Source: CAD feature listing. Evaluate the final solid. Frame: model axes, mm. Give positions to 0.01 mm unless a question says otherwise; leave off trailing zeros. Order: outer loops, then holes, each group sorted by start corner. A loop starts at its lowest first (then second) coordinate and runs counter-clockwise, first axis right, second up.
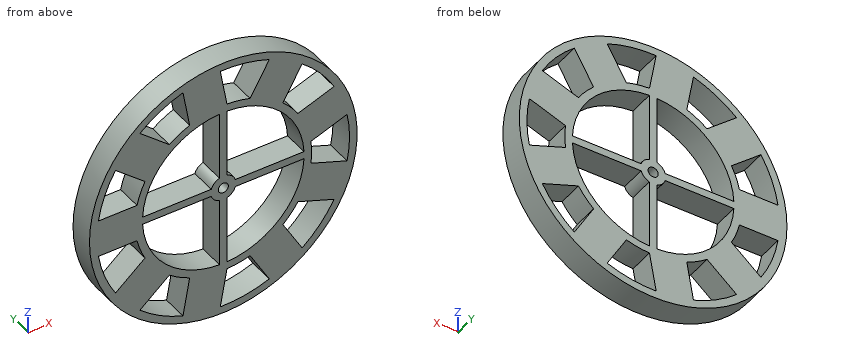
Autodesk Inventor part; units mm, degrees
ref_plane "YZ Plane" through (0, 0, 0) normal (1, 0, 0) x (0, 1, 0)
ref_plane "XZ Plane" through (0, 0, 0) normal (0, 1, 0) x (-1, 0, 0)
ref_plane "XY Plane" through (0, 0, 0) normal (0, 0, 1) x (1, 0, 0)
sketch "Sketch1" plane through (0, 0, 0) normal (0, 1, 0) x (-1, 0, 0)
  circle A0 centre (0, 0) radius 50
  circle A1 centre (0, 0) radius 35
  line L0 (49.4343, 7.5) -> (34.187, 7.5)
  line L1 (49.4343, -7.5) -> (34.187, -7.5)
  line L2 (41.8106, 7.5) -> (41.8106, -7.5) construction
  circle A2 centre (0, 0) radius 32
  line L3 (34.187, 7.5) -> (34.187, -7.5)
  line L4 (49.4343, 7.5) -> (49.4343, -7.5)
  line L5 (21.3678, 27.7203) -> (31.0097, 16.2296)
  line L6 (42.6898, 26.0304) -> (31.0097, 16.2296)
  line L7 (33.048, 37.5211) -> (42.6898, 26.0304)
  line L8 (33.048, 37.5211) -> (21.3678, 27.7203)
  line L9 (-1.4496, 34.97) -> (13.3226, 32.3652)
  line L10 (15.9702, 47.3809) -> (13.3226, 32.3652)
  line L11 (1.1981, 49.9856) -> (15.9702, 47.3809)
  line L12 (1.1981, 49.9856) -> (-1.4496, 34.97)
  line L13 (-23.5887, 25.8568) -> (-10.5983, 33.3568)
  line L14 (-18.222, 46.5614) -> (-10.5983, 33.3568)
  line L15 (-31.2123, 39.0614) -> (-18.222, 46.5614)
  line L16 (-31.2123, 39.0614) -> (-23.5887, 25.8568)
  line L17 (-34.6904, 4.6449) -> (-29.5601, 18.7403)
  line L18 (-43.8879, 23.9552) -> (-29.5601, 18.7403)
  line L19 (-49.0182, 9.8598) -> (-43.8879, 23.9552)
  line L20 (-49.0182, 9.8598) -> (-34.6904, 4.6449)
  line L21 (-29.5601, -18.7403) -> (-34.6904, -4.6449)
  line L22 (-49.0182, -9.8598) -> (-34.6904, -4.6449)
  line L23 (-43.8879, -23.9552) -> (-49.0182, -9.8598)
  line L24 (-43.8879, -23.9552) -> (-29.5601, -18.7403)
  line L25 (-10.5983, -33.3568) -> (-23.5887, -25.8568)
  line L26 (-31.2123, -39.0614) -> (-23.5887, -25.8568)
  line L27 (-18.222, -46.5614) -> (-31.2123, -39.0614)
  line L28 (-18.222, -46.5614) -> (-10.5983, -33.3568)
  line L29 (13.3226, -32.3652) -> (-1.4496, -34.97)
  line L30 (1.1981, -49.9856) -> (-1.4496, -34.97)
  line L31 (15.9702, -47.3809) -> (1.1981, -49.9856)
  line L32 (15.9702, -47.3809) -> (13.3226, -32.3652)
  line L33 (31.0097, -16.2296) -> (21.3678, -27.7203)
  line L34 (33.048, -37.5211) -> (21.3678, -27.7203)
  line L35 (42.6898, -26.0304) -> (33.048, -37.5211)
  line L36 (42.6898, -26.0304) -> (31.0097, -16.2296)
  circle A3 centre (0, 0) radius 53
  circle A4 centre (0, 0) radius 2
  circle A5 centre (0, 0) radius 5
  line L37 (1.5, -31.9648) -> (1.5, -4.7697)
  line L38 (-1.5, -31.9648) -> (-1.5, -4.7697)
  line L39 (1.5, -18.3673) -> (-1.5, -18.3673) construction
  line L40 (-31.9648, -1.5) -> (-4.7697, -1.5)
  line L41 (-4.7697, 1.5) -> (-31.9648, 1.5)
  line L42 (1.5, 31.9648) -> (1.5, 4.7697)
  line L43 (-1.5, 4.7697) -> (-1.5, 31.9648)
  line L44 (4.7697, -1.5) -> (31.9648, -1.5)
  line L45 (4.7697, 1.5) -> (31.9648, 1.5)
  line L46 (18.3673, -1.5) -> (18.3673, 1.5) construction
  line L47 (-1.5, 18.3673) -> (1.5, 18.3673) construction
  line L48 (-18.3673, 1.5) -> (-18.3673, -1.5) construction
  point P0 (41.8106, 0)
  point P1 (36.8497, 21.13)
  point P2 (27.2079, 32.6207)
  point P3 (14.6464, 39.8731)
  point P4 (-0.1257, 42.4778)
  point P5 (-14.4101, 39.9591)
  point P6 (-27.4005, 32.4591)
  point P7 (-36.724, 21.3478)
  point P8 (-41.8543, 7.2524)
  point P9 (-41.8543, -7.2524)
  point P10 (-36.724, -21.3478)
  point P11 (-27.4005, -32.4591)
  point P12 (-14.4101, -39.9591)
  point P13 (-0.1257, -42.4778)
  point P14 (14.6464, -39.8731)
  point P15 (27.2079, -32.6207)
  point P16 (36.8497, -21.13)
  point P17 (0, -18.3673)
  point P18 (-34.6904, -4.6449)
  dimension "d0" = 100
  dimension "d1" = 15
  dimension "d2" = 15
  dimension "d3" = 3
  dimension "d6" = 360
  dimension "d8" = 3
  dimension "d9" = 4
  dimension "d11" = 3
  dimension "d12" = 3
  dimension "d13" = 3
  dimension "d14" = 3
extrude "Extrusion1" add sketch "Sketch1" along normal blind 10 contours A0 L4 | L4 L1 A1 L0 | L7 A0 | L6 A1 L8 L7 | L3 A1 L33 L29 L25 L21 L17 L13 L9 L5 | A1 L3 | A0 L35 | L35 L34 A1 L36 | L5 A1 | A1 L33 | L11 A0 | L10 A1 L12 L11 | A0 L31 | L31 L30 A1 L32 | L9 A1 | A1 L29 | L15 A0 | L14 A1 L16 L15 | A0 L27 | L27 L26 A1 L28 | L13 A1 | A1 L25 | L19 A0 | L18 A1 L20 L19 | A0 L23 | L23 L22 A1 L24 | L17 A1 | A1 L21 | A2 L44 A5 L45 | L42 A5 L43 A2 | A5 | A2 L38 A5 L37 | L41 A5 L40 A2 | A3 | A4
hole "Hole1" at (0, 0, 0) direction (0, 1, 0) diameter 4 end through all
properties part number "Rueda_SENSORVEL_3DPrint"
1) Section query C-C on x = -19. Output: boundary loops of the cut face in (y, z), and give its area (3 significant figures).
Checks:
outline: (0, -49.48) - (10, -49.48) - (10, -46.25) - (0, -46.25) - close; (0, -29.39) - (10, -29.39) - (10, -25.75) - (0, -25.75) - close; (0, -1.5) - (10, -1.5) - (10, 1.5) - (0, 1.5) - close; (0, 25.75) - (10, 25.75) - (10, 29.39) - (0, 29.39) - close; (0, 46.25) - (10, 46.25) - (10, 49.48) - (0, 49.48) - close
area: 167 mm2
2) Section query B-B on z = -12. Output: boundary loops of the cut face in (x, y).
Checks:
outline: (-51.62, 0) - (-48.54, 0) - (-48.54, 10) - (-51.62, 10) - close; (-32.88, 0) - (-29.66, 0) - (-29.66, 10) - (-32.88, 10) - close; (-1.5, 0) - (1.5, 0) - (1.5, 10) - (-1.5, 10) - close; (29.66, 0) - (51.62, 0) - (51.62, 10) - (29.66, 10) - close
3) Ray query, L1, parallel to X at y = 8.75, z = -29.5; L2, parallel to X at y = 6.75, z = -14; L3, parallel to X at y = 3.75, z = -43. Return the intervals inside material, ascending.
Checks:
L1: x = -44.03 to -23.49, -18.83 to -12.4, -1.5 to 1.5, 12.4 to 25.69, 40.37 to 44.03
L2: x = -51.12 to -48, -32.08 to -28.77, -1.5 to 1.5, 28.77 to 51.12
L3: x = -30.98 to -25.51, -15.2 to 0.03, 16.17 to 30.98
4) First-contact query: pin 1 Ø3 at (y, z) = (7.5, 16.5) entering from +X; pin 2 Ø5 at (x, y) = (-40.5, 7) entering from -Z; pin 3 Ø5 at (y, z) = (5.5, -22.5) entering from +X. Flat tips, straight axial feed; report the tip coordinate or a pass-through.
Checks:
pin 1: stops at x = 50.83
pin 2: stops at z = -36.95
pin 3: stops at x = 49.08
5) Section query D-D on y = 2.25. State how many separate pieces and enclosed holes the cut face has, and give its area (3 significant figures).
Checks:
separate pieces: 1
enclosed holes: 14
area: 4,030 mm2
6) Section query A-A on z = -41. Output: boundary loops of the cut face in (x, y).
Checks:
outline: (-33.59, 0) - (-28.62, 0) - (-28.62, 10) - (-33.59, 10) - close; (-14.85, 0) - (0.39, 0) - (0.39, 10) - (-14.85, 10) - close; (15.01, 0) - (33.59, 0) - (33.59, 10) - (15.01, 10) - close
